Part model, mm, in its own coordinate system. A direction names the side the tool comes from. Round coordinates to 2 decimals unless told otherwise and drop trailing zeros. Loops run counter-clockwise (first coordinate to the right, second up) from the corner with the lowest first, then second, coordinate; pieces in that order, holes last. Notation, with made-up numbers: M 44.5,71.5 L 81.5,71.5 A25 ccw 81.5,88.5 Z; hole C 4,-2 d4. An arc over 180 degrees is marked long. Put each result on its own line as item: value. Start each with the question number.
1) Slice it at B-B on z = 27. Give the cut face in (x, y), then the cut area to 3 significant figures.
2) Which spindle directions (+Z, -Z, +X, -X, +Y, -Y) get a long thin tool onto all of the face, cutting with end or side? Do faces 1 (the flat face through (0, -9, 35)), 2 (the flat face through (0, 20.7, 28)), 3 (the flat face through (13, 44, 22)). Say none if no direction does.
3) Slice it at A-A on y = 7.5. Give the cut face in (x, z), then the cut area to 3 significant figures.
4) Drop flat-ended pins along their axis: pin 1 Ø13.5 at (x, y) = (11.5, -7.5) entering from +Z; pin 2 Ø11.5 at (x, z) = (2, 14) entering from +Y; pin 3 Ø4 at (x, y) = (3.5, 23) entering from +Z. Give the stop position or say it passes through.
5) Pull direction X, two halves, no side cores. Call faces 4 (the cylindrical face through (-1.846, -7.944, 55.549)), 5 (the flat face through (0, 12, 52)), 6 (the flat face through (9.5, 40, 28)): +X half, -X half, draft (parallel to the pull), parting line (faces both ways), or undercut.
6) Probe line 1 along Z through (x, y) = (7.5, -9); line 2 along Z through (x, y) = (3, 8.5); line 3 along X through (y, z) = (-1, 26). List the from-to ranges inside material, lowest first.
```python
from build123d import *

# Parameters (mm, degrees)
SKETCH4_W            = 31.4
SKETCH4_H            = 31.4
SKETCH4_W_2          = 25.4
SKETCH4_H_2          = 25.4
BOSS_EXTRUDE3_DEPTH  = 30
SKETCH5_W            = 31.4
SKETCH5_H            = 31.4
BOSS_EXTRUDE4_DEPTH  = 5
SKETCH6_W            = 31.4
SKETCH6_H            = 8
BOSS_EXTRUDE5_DEPTH  = 5
BOSS_EXTRUDE6_DEPTH  = 8
SKETCH8_R            = 4
BOSS_EXTRUDE7_DEPTH  = 8
SKETCH9_W            = 31.4
SKETCH9_H            = 10
BOSS_EXTRUDE8_DEPTH  = 5
SKETCH10_W           = 31.4
SKETCH10_H           = 10
BOSS_EXTRUDE9_DEPTH  = 13
SKETCH11_W           = 6.2
SKETCH11_H           = 10
BOSS_EXTRUDE10_DEPTH = 40
BOSS_EXTRUDE11_DEPTH = 3
SKETCH13_W           = 31.4
SKETCH13_H           = 31.4
CUT_EXTRUDE1_DEPTH   = 31.4
SKETCH15_R           = 4
BOSS_EXTRUDE12_DEPTH = 8
SKETCH16_W           = 31.4
SKETCH16_H           = 13
BOSS_EXTRUDE13_DEPTH = 4.6
SKETCH17_W           = 31.4
SKETCH17_H           = 3.6
BOSS_EXTRUDE14_DEPTH = 0.6
CUT_EXTRUDE2_DEPTH   = 3.6


with BuildPart() as part:
    # Sketch4 → Boss-Extrude3 (new body)
    with BuildSketch(Plane.XY):
        Rectangle(SKETCH4_W, SKETCH4_H)
        Rectangle(SKETCH4_W_2, SKETCH4_H_2, mode=Mode.SUBTRACT)
    extrude(amount=BOSS_EXTRUDE3_DEPTH)

    # Sketch5 → Boss-Extrude4 (add)
    with BuildSketch(Plane.XY.offset(30)):
        Rectangle(SKETCH5_W, SKETCH5_H)
    extrude(amount=BOSS_EXTRUDE4_DEPTH)

    # Sketch6 → Boss-Extrude5 (add)
    with BuildSketch(Plane.XY.offset(35)):
        Rectangle(SKETCH6_W, SKETCH6_H)
    extrude(amount=BOSS_EXTRUDE5_DEPTH)

    # Sketch7 → Boss-Extrude6 (add)
    with BuildSketch(Plane.XZ.offset(4)):
        with BuildLine():
            Line((-15.7, 40), (-15.7, 52))
            ThreePointArc((-15.7, 52), (-11.306601718, 62.606601718), (-0.7, 67))
            Line((-0.7, 67), (0.7, 67))
            ThreePointArc((0.7, 67), (11.306601718, 62.606601718), (15.7, 52))
            Line((15.7, 52), (15.7, 40))
            Line((15.7, 40), (-15.7, 40))
        make_face()
    extrude(amount=-BOSS_EXTRUDE6_DEPTH)

    # Sketch8 → Boss-Extrude7 (add)
    with BuildSketch(Plane.XZ.offset(4)):
        with Locations(Location((0, 52, 0), (0, 0, 180))):
            Circle(SKETCH8_R)
    boss_extrude7 = extrude(amount=BOSS_EXTRUDE7_DEPTH)

    # Mirror1: Boss-Extrude7 across plane
    add(boss_extrude7.mirror(Plane.ZX))

    # Sketch9 → Boss-Extrude8 (add)
    with BuildSketch(Plane(origin=(0, 15.7, 0), x_dir=(1, 0, 0), z_dir=(0, 1, 0))):
        with Locations((0, -27)):
            Rectangle(SKETCH9_W, SKETCH9_H)
    extrude(amount=BOSS_EXTRUDE8_DEPTH)

    # Sketch10 → Boss-Extrude9 (add)
    with BuildSketch(Plane(origin=(0, 15.7, 0), x_dir=(1, 0, 0), z_dir=(0, 1, 0))):
        with Locations((0, -17)):
            Rectangle(SKETCH10_W, SKETCH10_H)
    extrude(amount=BOSS_EXTRUDE9_DEPTH)

    # Sketch11 → Boss-Extrude10 (add)
    with BuildSketch(Plane(origin=(0, 20.7, 0), x_dir=(1, 0, 0), z_dir=(0, 1, 0))):
        with Locations((-12.6, -27)):
            Rectangle(SKETCH11_W, SKETCH11_H)
        with Locations((12.6, -27)):
            Rectangle(SKETCH11_W, SKETCH11_H)
    extrude(amount=BOSS_EXTRUDE10_DEPTH)

    # Sketch12 → Boss-Extrude11 (add)
    with BuildSketch(Plane.XY.offset(32)):
        Polygon((-15.7, 60.7), (-9.5, 60.7), (-9.5, 20.7), (9.5, 20.7), (9.5, 60.7), (15.7, 60.7), (15.7, 15.7), (-15.7, 15.7), align=None)
    extrude(amount=BOSS_EXTRUDE11_DEPTH)

    # Sketch13 → Cut-Extrude1 (cut)
    with BuildSketch(Plane.ZY.offset(15.7)):
        with Locations((15.7, 0)):
            Rectangle(SKETCH13_W, SKETCH13_H)
    extrude(amount=-CUT_EXTRUDE1_DEPTH, mode=Mode.SUBTRACT)

    # Sketch15 → Boss-Extrude12 (add)
    with BuildSketch(Plane(origin=(0, 0, 31.4), x_dir=(-1, 0, 0), z_dir=(0, 0, -1))):
        with BuildLine():
            Line((15.7, -1.3), (15.7, 15.7))
            Line((15.7, 15.7), (-15.7, 15.7))
            Line((-15.7, 15.7), (-15.7, -1.3))
            ThreePointArc((-15.7, -1.3), (-11.306601718, -11.906601718), (-0.7, -16.3))
            Line((-0.7, -16.3), (0.7, -16.3))
            ThreePointArc((0.7, -16.3), (11.306601718, -11.906601718), (15.7, -1.3))
        make_face()
        with Locations(Location((0, -1.3, 0), (0, 0, 90))):
            Circle(SKETCH15_R, mode=Mode.SUBTRACT)
    boss_extrude12 = extrude(amount=BOSS_EXTRUDE12_DEPTH)

    # Mirror2: Boss-Extrude12 across plane
    add(boss_extrude12.mirror(Plane(origin=(0, 0, 19.4), x_dir=(1, 0, 0), z_dir=(0, 0, -1))))

    # Sketch16 → Boss-Extrude13 (add)
    with BuildSketch(Plane(origin=(0, 0, 12), x_dir=(-1, 0, 0), z_dir=(0, 0, -1))):
        with Locations((0, 22.2)):
            Rectangle(SKETCH16_W, SKETCH16_H)
    extrude(amount=BOSS_EXTRUDE13_DEPTH)

    # Sketch17 → Boss-Extrude14 (add)
    with BuildSketch(Plane.XZ.offset(15.7)):
        with Locations((0, 33.2)):
            Rectangle(SKETCH17_W, SKETCH17_H)
    extrude(amount=BOSS_EXTRUDE14_DEPTH)

    # Sketch24 → Cut-Extrude2 (cut)
    with BuildSketch(Plane(origin=(0, 0, 31.4), x_dir=(-1, 0, 0), z_dir=(0, 0, -1))):
        with BuildLine():
            Line((-15.7, -3.955876224), (-15.7, -16.3))
            Line((-15.7, -16.3), (-0.7, -16.3))
            ThreePointArc((-0.7, -16.3), (-10.301298901, -12.800983891), (-15.399984201, -3.944829955))
            Line((-15.399984201, -3.944829955), (-15.7, -3.955876224))
        make_face()
    cut_extrude2 = extrude(amount=-CUT_EXTRUDE2_DEPTH, mode=Mode.SUBTRACT)

    # Mirror3: Cut-Extrude2 across plane
    add(cut_extrude2.mirror(Plane(origin=(0, 0, 0), x_dir=(0, 0, 1), z_dir=(1, 0, 0))), mode=Mode.SUBTRACT)


solid = part.part
```
Recorded:
1. outline: M -15.7,-1.3 A15 ccw -0.7,-16.3 L 0.7,-16.3 A15 ccw 15.7,-1.3 L 15.7,60.7 L 9.5,60.7 L 9.5,20.7 L -9.5,20.7 L -9.5,60.7 L -15.7,60.7 Z; hole C 0,-1.3 d8
1. area: 1,510 mm2
2. face 1: +X, -X, -Y
2. face 2: +Z, +Y
2. face 3: -Z, +X, -X, +Y
3. outline: M -15.7,7.4 L 15.7,7.4 L 15.7,15.4 L -15.7,15.4 Z; M -15.7,23.4 L 15.7,23.4 L 15.7,35 L -15.7,35 Z; C 0,52 d8
3. area: 666 mm2
4. pin 1: stops at z = 66.13
4. pin 2: stops at y = 28.7
4. pin 3: stops at z = 22
5. face 4: parting line
5. face 5: draft
5. face 6: undercut
6. line 1: z = 7.4 to 15.4, 23.4 to 35
6. line 2: z = 7.4 to 15.4, 23.4 to 35, 49.35 to 54.65
6. line 3: x = -15.7 to -3.99, 3.99 to 15.7
